```python
from build123d import *

# Parameters (mm, degrees)
SKETCH1_R           = 1.25
BOSS_EXTRUDE4_DEPTH = 4
FILLET1_R           = 10
SKETCH2_R           = 1.25
BOSS_EXTRUDE5_DEPTH = 1.2
SKETCH3_R           = 1.25
BOSS_EXTRUDE6_DEPTH = 1.2


with BuildPart() as part:
    # Sketch1 → Boss-Extrude4 (new body)
    with BuildSketch(Plane.XY):
        Polygon((-9.75, 9.75), (-9.75, 0), (-9.75, -9.75), (29.5, -9.75), (29.5, -6.75), (29.5, 6.75), (29.5, 9.75), align=None)
        with Locations((14.5, -6.75)):
            Circle(SKETCH1_R, mode=Mode.SUBTRACT)
        with BuildLine():
            ThreePointArc((4.901044183, -6.003521127), (-3.322604971, -7.001628111), (-7.75, 0))
            ThreePointArc((-7.75, 0), (-3.322604971, 7.001628111), (4.901044183, 6.003521127))
            ThreePointArc((4.901044183, 6.003521127), (7.868246727, 4.330212616), (11.22497216, 3.75))
            Line((11.22497216, 3.75), (23.75, 3.75))
            ThreePointArc((23.75, 3.75), (26.401650429, 2.651650429), (27.5, 0))
            ThreePointArc((27.5, 0), (26.401650429, -2.651650429), (23.75, -3.75))
            Line((23.75, -3.75), (11.22497216, -3.75))
            ThreePointArc((11.22497216, -3.75), (7.868246727, -4.330212616), (4.901044183, -6.003521127))
        make_face(mode=Mode.SUBTRACT)
        with Locations((14.5, 6.75)):
            Circle(SKETCH1_R, mode=Mode.SUBTRACT)
    extrude(amount=BOSS_EXTRUDE4_DEPTH)

    # Fillet1
    # the kernel refuses this fillet: 10 mm, written as the material it takes off along each edge
    with BuildSketch(Plane(origin=(-9.75, -9.75, -25), x_dir=(0, 1, 0), z_dir=(0, 0, 1))) as fillet1_piece_1:
        with BuildLine():
            CenterArc((FILLET1_R, -FILLET1_R), FILLET1_R, 90, 90)
            Line((0, -FILLET1_R), (0, 0))
            Line((0, 0), (FILLET1_R, 0))
        make_face()
    extrude(amount=54, mode=Mode.SUBTRACT)
    with BuildSketch(Plane(origin=(-9.75, 9.75, -25), x_dir=(0, -1, 0), z_dir=(0, 0, 1))) as fillet1_piece_2:
        with BuildLine():
            CenterArc((FILLET1_R, FILLET1_R), FILLET1_R, 180, 90)
            Line((0, FILLET1_R), (0, 0))
            Line((0, 0), (FILLET1_R, 0))
        make_face()
    extrude(amount=54, mode=Mode.SUBTRACT)

    # Sketch2 → Boss-Extrude5 (add)
    # profile 1 of 4: a face of its own
    with BuildSketch(Plane.XY.offset(4)):
        with BuildLine():
            ThreePointArc((8.882472313, 4.028236041), (5.388428188, 8.129565896), (0.25, 9.75))
            ThreePointArc((0.25, 9.75), (-6.732120022, 6.908910532), (-9.746874512, 0))
            ThreePointArc((-9.746874512, 0), (-6.957195545, -6.682267477), (-0.388423062, -9.729599992))
            Line((-0.388423062, -9.729599992), (0.667724562, -9.730320853))
            ThreePointArc((0.667724562, -9.730320853), (5.561475334, -8.012177738), (8.882472313, -4.028236041))
            ThreePointArc((8.882472313, -4.028236041), (6.780629621, -4.791885277), (4.901044183, -6.003521127))
            ThreePointArc((4.901044183, -6.003521127), (-7.75, 0), (4.901044183, 6.003521127))
            ThreePointArc((4.901044183, 6.003521127), (6.780629621, 4.791885277), (8.882472313, 4.028236041))
        make_face()
    # profile 2 of 4: a face of its own
    with BuildSketch(Plane.XY.offset(4)):
        with BuildLine():
            ThreePointArc((9.753204602, 0), (9.5330365, 2.060634631), (8.882472313, 4.028236041))
            ThreePointArc((8.882472313, 4.028236041), (6.780629621, 4.791885277), (4.901044183, 6.003521127))
            ThreePointArc((4.901044183, 6.003521127), (-7.75, 0), (4.901044183, -6.003521127))
            ThreePointArc((4.901044183, -6.003521127), (6.780629621, -4.791885277), (8.882472313, -4.028236041))
            ThreePointArc((8.882472313, -4.028236041), (9.5330365, -2.060634631), (9.753204602, 0))
        make_face()
        Circle(SKETCH2_R, mode=Mode.SUBTRACT)
    # profile 3 of 4: a face of its own
    with BuildSketch(Plane.XY.offset(4)):
        with BuildLine():
            Line((29.5, -9.75), (29.5, 9.75))
            Line((29.5, 9.75), (0.25, 9.75))
            ThreePointArc((0.25, 9.75), (5.388428188, 8.129565896), (8.882472313, 4.028236041))
            ThreePointArc((8.882472313, 4.028236041), (10.045489135, 3.819802631), (11.22497216, 3.75))
            Line((11.22497216, 3.75), (23.75, 3.75))
            ThreePointArc((23.75, 3.75), (27.5, 0), (23.75, -3.75))
            Line((23.75, -3.75), (11.22497216, -3.75))
            ThreePointArc((11.22497216, -3.75), (10.045489135, -3.819802631), (8.882472313, -4.028236041))
            ThreePointArc((8.882472313, -4.028236041), (5.561475334, -8.012177738), (0.667724562, -9.730320853))
            Line((0.667724562, -9.730320853), (29.5, -9.75))
        make_face()
        with Locations((14.5, -6.75)):
            Circle(SKETCH2_R, mode=Mode.SUBTRACT)
        with Locations((14.5, 6.75)):
            Circle(SKETCH2_R, mode=Mode.SUBTRACT)
    # profile 4 of 4: a face of its own
    with BuildSketch(Plane.XY.offset(4)):
        with BuildLine():
            ThreePointArc((11.22497216, 3.75), (10.045489135, 3.819802631), (8.882472313, 4.028236041))
            ThreePointArc((8.882472313, 4.028236041), (9.5330365, 2.060634631), (9.753204602, 0))
            ThreePointArc((9.753204602, 0), (9.5330365, -2.060634631), (8.882472313, -4.028236041))
            ThreePointArc((8.882472313, -4.028236041), (10.045489135, -3.819802631), (11.22497216, -3.75))
            Line((11.22497216, -3.75), (23.75, -3.75))
            ThreePointArc((23.75, -3.75), (27.5, 0), (23.75, 3.75))
            Line((23.75, 3.75), (11.22497216, 3.75))
        make_face()
        with Locations((23.75, 0)):
            Circle(SKETCH2_R, mode=Mode.SUBTRACT)
    extrude(amount=BOSS_EXTRUDE5_DEPTH)

    # Sketch3 → Boss-Extrude6 (add)
    # profile 1 of 2: a face of its own
    with BuildSketch(Plane.XY.offset(5.2)):
        with BuildLine():
            ThreePointArc((9.75, 0), (6.938066581, 6.850235917), (0.124208797, 9.749208797))
            ThreePointArc((0.124208797, 9.749208797), (-6.777009203, 6.864853594), (-9.746874512, 0))
            ThreePointArc((-9.746874512, 0), (-6.957195545, -6.682267477), (-0.388423062, -9.729599992))
            Line((-0.388423062, -9.729599992), (0.619672772, -9.730288056))
            ThreePointArc((0.619672772, -9.730288056), (7.110003851, -6.671607395), (9.75, 0))
        make_face()
        Circle(SKETCH3_R, mode=Mode.SUBTRACT)
    # profile 2 of 2: a face of its own
    with BuildSketch(Plane.XY.offset(5.2)):
        with BuildLine():
            Line((29.5, 9.75), (0.25, 9.75))
            ThreePointArc((0.25, 9.75), (0.187103155, 9.749802197), (0.124208797, 9.749208797))
            ThreePointArc((0.124208797, 9.749208797), (6.938066581, 6.850235917), (9.75, 0))
            ThreePointArc((9.75, 0), (7.110003851, -6.671607395), (0.619672772, -9.730288056))
            Line((0.619672772, -9.730288056), (29.5, -9.75))
            Line((29.5, -9.75), (29.5, 9.75))
        make_face()
        with Locations((14.5, -6.75)):
            Circle(SKETCH3_R, mode=Mode.SUBTRACT)
        with Locations((23.75, 0)):
            Circle(SKETCH3_R, mode=Mode.SUBTRACT)
        with Locations((14.5, 6.75)):
            Circle(SKETCH3_R, mode=Mode.SUBTRACT)
    extrude(amount=BOSS_EXTRUDE6_DEPTH)


solid = part.part
```
Input: part model. Units: mm. Frame: model coordinates. A direction names the side the tool comes from. Give positions to 0.01 mm unless a question says otherwise; leave off trailing zeros. Order: outer loops, then holes, each group sorted by start corner. A loop starts at its lowest first (then second) coordinate and runs counter-clockwise, first axis right, second up. Notation, with made-up numbers: M 45.5,-38.75 L 61.5,-38.75 A17 ccw 61.5,-32.75 Z; hole C 38,-4 d1. An arc over 180 degrees is marked long. Return JSON: item names as keys, results as strings.
Item 1: Ray query, probe 1 along Y at (x, z) = (14.5, 2.75); probe 2 along Y at (x, z) = (14.5, 4.75); probe 3 along X at (y, z) = (-5.75, 1.5). Return the intervals inside material, ascending.
Solutions:
{"probe 1": "-9.75 to -8, -5.5 to -3.75, 3.75 to 5.5, 8 to 9.75", "probe 2": "-9.74 to -8, -5.5 to 5.5, 8 to 9.75", "probe 3": "-7.75 to -5.2, 5.22 to 13.75, 15.25 to 29.5"}
Item 2: Access query for faces 1 (the flat face through (17, 3.75, 2)), 2 (the cylindrical face through (25, 0, 5)). Directions: +Z, -Z, +X, -X, +Y, -Y. A direction counts if a zero-diameter tool reaches every point of the face in a straight line with its end or side. Return the directions, or none.
Solutions:
{"face 1": "-Z", "face 2": "+Z, -Z"}
Item 3: Cut plane B-B (y = 6.75). Return loops of the section in (x, z), then the cut area to 3 significant figures.
Solutions:
{"outline": "M -6.89,0 L -3.81,0 L -3.81,4 L 3.81,4 L 3.81,0 L 13.25,0 L 13.25,6.4 L -6.89,6.4 Z; M 15.75,0 L 29.5,0 L 29.5,6.4 L 15.75,6.4 Z", "area": "186 mm^2"}
Item 4: Cut plane A-A (x = 14.5). State how many separate pieces and enclosed holes the cut face has, then the cut area to 3 significant figures.
Solutions:
{"separate pieces": "3", "enclosed holes": "0", "area": "62.8 mm^2"}
Item 5: First-contact query: P1, Ø4, axis at x = 23.75, y = 0, coming from the -Z side; P2, Ø2, axis at x = 0, z = 1, coming from the +Y side; P3, Ø1.5, axis at x = 14.5, y = -6.75, coming from the +Z side; P4, Ø1, axis at x = -2, z = 5, coming from the -Y side. Flat tips, straight axial feed; report the tip coordinate or a pass-through.
Solutions:
{"P1": "z = 4", "P2": "y = 9.75", "P3": "through", "P4": "y = -9.6"}
Item 6: Pull-direction query (X, two-part tool) for faces 3 (the cylindrical face through (-6.81, -6.83, 3.16)), 4 (the flat face through (18, -3.75, 2)), 5 (the flat face through (15, 9.75, 3)), 6 (the flat face through (10, 0, 4)); classes: +X half, -X half, draft (parallel to the pull), parting line (faces both ways), or undercut.
Solutions:
{"face 3": "-X half", "face 4": "undercut", "face 5": "draft", "face 6": "undercut"}
Item 7: Cut plane D-D (y = -0.5). Return loops of the section in (x, z), then the cut area to 3 significant figures.
Solutions:
{"outline": "M -9.72,0 L -7.73,0 L -7.73,4 L -1.15,4 L -1.15,6.4 L -9.72,6.4 Z; M 1.15,4 L 22.6,4 L 22.6,6.4 L 1.15,6.4 Z; M 24.9,4 L 27.47,4 L 27.47,0 L 29.5,0 L 29.5,6.4 L 24.9,6.4 Z", "area": "99.2 mm^2"}
Item 8: Cut plane C-C (z = 2.5). Return loops of the section in (x, y), then the cut area to 3 significant figures.
Solutions:
{"outline": "M -9.75,0 A10 ccw 0.25,-9.75 L 29.5,-9.75 L 29.5,9.75 L 0.25,9.75 A10 ccw Z; hole M 4.9,-6 A10 cw 11.22,-3.75 L 23.75,-3.75 A3.75 ccw 23.75,3.75 L 11.22,3.75 A10 cw 4.9,6 A7.75 ccw long Z; hole C 14.5,-6.75 d2.5; hole C 14.5,6.75 d2.5", "area": "375 mm^2"}
